The model under review builds one solid part; all positions refer to its coordinate system, in mm. A direction names the side the tool comes from. Round coordinates to 2 decimals unless told otherwise and drop trailing zeros. Loops run counter-clockwise (first coordinate to the right, second up) from the corner with the lowest first, then second, coordinate; pieces in that order, holes last. Notation, with made-up numbers: M 11.5,34 L 28.5,34 A25 ccw 28.5,55 Z; hole C 52,85 d3. An arc over 180 degrees is marked long. Answer in a Markdown table with one row per item. Add a question column.
from build123d import *

# Parameters (mm, degrees)
EXTRUDE1_DEPTH       = 40
EXTRUDE2_DEPTH       = 6.86
EXTRUDE3_DEPTH       = 38
SKETCH5_W            = 18.35
SKETCH5_H            = 67.74
EXTRUDE4_DEPTH       = 81.231512798
EXTRUDE4_DEPTH_BACK  = 12
SKETCH6_W            = 14.5
SKETCH6_H            = 67.74
EXTRUDE5_DEPTH       = 2
EXTRUDE6_DEPTH       = 83.825796222
EXTRUDE7_DEPTH       = 10.85
EXTRUDE8_DEPTH       = 10.85
SKETCH10_R           = 0.925
EXTRUDE9_DEPTH       = 82.005837077
EXTRUDE10_DEPTH      = 81.630364259
EXTRUDE10_DEPTH_BACK = 1.25
SKETCH12_W           = 3.2
SKETCH12_H           = 0.6
EXTRUDE11_DEPTH      = 0.2
EXTRUDE12_DEPTH      = 0.2


with BuildPart() as part:
    # Sketch1 → Extrude1 (new body)
    with BuildSketch(Plane.XY):
        Polygon((8.175, 0), (-8.175, 0), (-8.175, 2.5), (-10.325, 2.5), (-10.325, 15.7), (10.325, 15.7), (10.325, 2.5), (8.175, 2.5), align=None)
    extrude(amount=-EXTRUDE1_DEPTH)

    # Sketch2 → Extrude2 (add)
    with BuildSketch(Plane.XY):
        with BuildLine():
            Line((-8.825, 15.7), (8.825, 15.7))
            ThreePointArc((8.825, 15.7), (6.943835072, 17.710022023), (4.375, 18.7))
            Line((4.375, 18.7), (-4.375, 18.7))
            ThreePointArc((-4.375, 18.7), (-6.943835072, 17.710022023), (-8.825, 15.7))
        make_face()
    extrude(amount=-EXTRUDE2_DEPTH)

    # Sketch4 → Extrude3 (add)
    with BuildSketch(Plane(origin=(0, 0, -40), x_dir=(-1, 0, 0), z_dir=(0, 0, -1))):
        with BuildLine():
            Line((-10.325, 15.7), (-8.825, 15.7))
            add(Edge.make_bspline(
                [(-2.425, 14.6), (-5.625, 19.703568586), (-8.825, 15.7)],
                knots=[0, 0, 0, 1, 1, 1], degree=2))
            Line((-2.425, 14.6), (2.425, 14.6))
            add(Edge.make_bspline(
                [(2.425, 14.6), (5.625, 19.703568586), (8.825, 15.7)],
                knots=[0, 0, 0, 1, 1, 1], degree=2))
            Line((8.825, 15.7), (10.325, 15.7))
            Line((10.325, 15.7), (10.325, 2.5))
            Line((10.325, 2.5), (8.175, 2.5))
            Line((8.175, 2.5), (8.175, 0))
            Line((8.175, 0), (-8.175, 0))
            Line((-8.175, 0), (-8.175, 2.5))
            Line((-8.175, 2.5), (-10.325, 2.5))
            Line((-10.325, 2.5), (-10.325, 15.7))
        make_face()
    extrude(amount=EXTRUDE3_DEPTH)

    # Sketch5 → Extrude4 (cut, two sides)
    with BuildSketch(Plane(origin=(0, 15.7, 0), x_dir=(1, 0, 0), z_dir=(0, 1, 0))) as extrude4_sk:
        with Locations((0, 40.73)):
            Rectangle(SKETCH5_W, SKETCH5_H)
    extrude(amount=EXTRUDE4_DEPTH, mode=Mode.SUBTRACT)
    extrude(extrude4_sk.sketch, amount=-EXTRUDE4_DEPTH_BACK, mode=Mode.SUBTRACT)

    # Sketch6 → Extrude5 (cut)
    with BuildSketch(Plane(origin=(0, 3.7, 0), x_dir=(1, 0, 0), z_dir=(0, 1, 0))):
        with Locations((0, 40.73)):
            Rectangle(SKETCH6_W, SKETCH6_H)
    extrude(amount=-EXTRUDE5_DEPTH, mode=Mode.SUBTRACT)

    # Sketch7 → Extrude6 (cut, through all)
    with BuildSketch(Plane(origin=(10.325, 0, 0), x_dir=(0, 0, -1), z_dir=(1, 0, 0))):
        with BuildLine():
            Line((12.066317198, 15.7), (19, 15.7))
            ThreePointArc((19, 15.7), (20.5, 15.45), (21.837837838, 14.727027027))
            ThreePointArc((21.837837838, 14.727027027), (40, 8.5), (58.162162162, 14.727027027))
            ThreePointArc((58.162162162, 14.727027027), (59.5, 15.45), (61, 15.7))
            Line((61, 15.7), (67.933682802, 15.7))
            Line((67.933682802, 15.7), (67.933682802, 19.991069183))
            Line((67.933682802, 19.991069183), (12.066317198, 19.991069183))
            Line((12.066317198, 19.991069183), (12.066317198, 15.7))
        make_face()
    extrude(amount=-EXTRUDE6_DEPTH, mode=Mode.SUBTRACT)

    # Sketch8 → Extrude7 (add)
    with BuildSketch(Plane(origin=(0, 15.7, 0), x_dir=(1, 0, 0), z_dir=(0, 1, 0))):
        Polygon((10.325, 4.58), (10.325, 5.98), (11.325, 6.36), (11.325, 4.2), align=None)
        Polygon((11.325, 76.6), (10.325, 76.22), (10.325, 74.82), (11.325, 74.44), align=None)
    extrude(amount=-EXTRUDE7_DEPTH)

    # Sketch9 → Extrude8 (cut)
    with BuildSketch(Plane(origin=(0, 15.7, 0), x_dir=(1, 0, 0), z_dir=(0, 1, 0))):
        Polygon((-10.325000262, 76.22), (-9.325000262, 76.6), (-9.325000262, 74.44), (-10.325000468, 74.82), align=None)
        Polygon((-10.325000787, 5.98), (-9.325000787, 6.36), (-9.325000787, 4.2), (-10.325000603, 4.58), align=None)
    extrude(amount=-EXTRUDE8_DEPTH, mode=Mode.SUBTRACT)

    # Sketch10 → Extrude9 (cut, through all)
    with BuildSketch(Plane.XZ):
        with Locations(Location((-5.45, -22.675, 0), (0, 0, 270))):
            Circle(SKETCH10_R)
        with Locations(Location((-5.45, -57.275, 0), (0, 0, 270))):
            Circle(SKETCH10_R)
        with Locations(Location((5.45, -57.275, 0), (0, 0, 90))):
            Circle(SKETCH10_R)
        with Locations(Location((5.45, -22.675, 0), (0, 0, 90))):
            Circle(SKETCH10_R)
    extrude(amount=-EXTRUDE9_DEPTH, mode=Mode.SUBTRACT)

    # Sketch11 → Extrude10 (cut, two sides)
    with BuildSketch(Plane(origin=(0, 1.7, 0), x_dir=(1, 0, 0), z_dir=(0, 1, 0))) as extrude10_sk:
        Polygon((-3.140598923, 57.275), (-4.295299462, 59.275), (-6.604700538, 59.275), (-7.759401077, 57.275), (-6.604700538, 55.275), (-4.295299462, 55.275), align=None)
        Polygon((3.140598923, 57.275), (4.295299462, 55.275), (6.604700538, 55.275), (7.759401077, 57.275), (6.604700538, 59.275), (4.295299462, 59.275), align=None)
        Polygon((-3.140598923, 22.675), (-4.295299462, 24.675), (-6.604700538, 24.675), (-7.759401077, 22.675), (-6.604700538, 20.675), (-4.295299462, 20.675), align=None)
        Polygon((3.140598923, 22.675), (4.295299462, 20.675), (6.604700538, 20.675), (7.759401077, 22.675), (6.604700538, 24.675), (4.295299462, 24.675), align=None)
    extrude(amount=EXTRUDE10_DEPTH, mode=Mode.SUBTRACT)
    extrude(extrude10_sk.sketch, amount=-EXTRUDE10_DEPTH_BACK, mode=Mode.SUBTRACT)

    # Sketch12 → Extrude11 (add)
    with BuildSketch(Plane(origin=(0, 18.7, 0), x_dir=(1, 0, 0), z_dir=(0, 1, 0))):
        with Locations((0, 4.853640731)):
            Rectangle(SKETCH12_W, SKETCH12_H)
    extrude(amount=EXTRUDE11_DEPTH)

    # Sketch13 → Extrude12 (add)
    with BuildSketch(Plane(origin=(0, 14.6, 0), x_dir=(1, 0, 0), z_dir=(0, 1, 0))):
        Polygon((-0.3, 77.7), (0.3, 77.7), (0.295752896, 76.599999935), (1.395761159, 76.599999935), (1.395761159, 75.999999935), (0.295752896, 75.999999935), (0.291472262, 74.9), (-0.308527738, 74.9), (-0.304247104, 75.999999935), (-1.404255368, 75.999999935), (-1.404255368, 76.599999935), (-0.304247104, 76.599999935), align=None)
    extrude(amount=EXTRUDE12_DEPTH)


solid = part.part
1. For pin 1 Ø0.8 at (x, z) = (-9.5, -75.5) entering from +Y; pin 2 Ø6 at (x, z) = (-5, -47) entering from +Y; pin 3 Ø2 at (y, z) = (3, -64.5) entering from +X (3 decimals), all flat-tipped, find the tip position at first contact; note any pin that passes through.
2. Machinability: for faces 1 (the flat face through (11.325, 10, -5)), 2 (the flat face through (-5, 1, -59.275)), 3 (the flat face through (9, 2.5, -38)), 4 (the flat face through (-10, 15.7, -69)), which of the approach directions +Z, -Z, +X, -X, +Y, -Y give a long, thin tool a straight path to every point of the face, cutting with its end or side? Answer none if there is none.
3. Mouldability with a two-part tool opening along Z and no side actions: class faces 5 (the flat face through (-7.25, 3, -14)), 6 (the flat face through (8.175, 1, -38)) as released by +Z, released by -Z, zero draft, split by the parting line, or undercut.
4. To check wall thickness, follow probe 1 along Z at (x, y) = (5.45, 0.35); probe 2 along Z at (x, y) = (5.25, 8.75); probe 3 along X at (y, z) = (7.25, -52.5) (3 decimals). State the ranges of each line that lie inside material, in increasing order.
5. Take a section at C-C, the plane x = 5.45. State how many separate pieces and enclosed holes the cut face has, and give its area (3 significant figures).
6. Take a section at B-B, the plane z = -49.5. State the section outline as (x, y) points (3 decimals).
Check sheet entries:
| question | item | result |
|---|---|---|
| 1 | pin 1 | stops at y = 15.7 |
| 1 | pin 2 | stops at y = 3.7 |
| 1 | pin 3 | stops at x = 10.325 |
| 2 | face 1 | +Z, -Z, +X, +Y, -Y |
| 2 | face 2 | +Y |
| 2 | face 3 | +Z, -Z, +X, -Y |
| 2 | face 4 | +Z, -Z, -X, +Y |
| 3 | face 5 | undercut |
| 3 | face 6 | zero draft |
| 4 | probe 1 | z = -78 to -58.2, -56.35 to -23.6, -21.75 to 0 |
| 4 | probe 2 | z = -78 to -74.6, -6.86 to 0 |
| 4 | probe 3 | x = -10.325 to -9.175, 9.175 to 10.325 |
| 5 | separate pieces | 3 |
| 5 | enclosed holes | 0 |
| 5 | area | 289 mm^2 |
| 6 | outline | M -10.325,2.5 L -8.175,2.5 L -8.175,0 L 8.175,0 L 8.175,2.5 L 10.325,2.5 L 10.325,10.066 L 9.175,10.066 L 9.175,3.7 L 7.25,3.7 L 7.25,1.7 L -7.25,1.7 L -7.25,3.7 L -9.175,3.7 L -9.175,10.066 L -10.325,10.066 Z |
